Autodesk Inventor part; units mm, degrees
ref_plane "YZ Plane" through (0, 0, 0) normal (1, 0, 0) x (0, 1, 0)
ref_plane "XZ Plane" through (0, 0, 0) normal (0, 1, 0) x (-1, 0, 0)
ref_plane "XY Plane" through (0, 0, 0) normal (0, 0, 1) x (1, 0, 0)
sketch "Esquisse1" plane through (0, 0, 0) normal (0, 1, 0) x (-1, 0, 0)
  circle A0 centre (-0.3398, 0) radius 22.5
  circle A1 centre (-0.3398, 0) radius 10
  line L0 (3.1602, 9.3675) -> (-3.8398, 9.3675)
  line L1 (-3.8398, 9.3675) -> (-3.8398, 30.3675)
  line L2 (-3.8398, 30.3675) -> (3.1602, 30.3675)
  line L3 (3.1602, 30.3675) -> (3.1602, 9.3675)
  line L4 (-8.8398, 35.3675) -> (-8.8398, 4.3675)
  line L5 (-8.8398, 4.3675) -> (8.1602, 4.3675)
  line L6 (8.1602, 4.3675) -> (8.1602, 35.3675)
  line L7 (8.1602, 35.3675) -> (-8.8398, 35.3675)
  line L8 (17.1996, -3) -> (9.1996, -3)
  line L9 (9.1996, -3) -> (9.1996, 3)
  line L10 (9.1996, 3) -> (17.1996, 3)
  line L11 (17.1996, 3) -> (17.1996, -3)
  line L12 (15.5701, 15.9099) -> (-16.2497, -15.9099) construction
  line L13 (-0.3398, -15.9099) -> (-16.2497, -15.9099) construction
  line L14 (-16.2497, -15.9099) -> (-16.2497, 0) construction
  line L15 (-0.3398, -15.9099) -> (-0.3398, 0) construction
  line L16 (-0.3398, 0) -> (-16.2497, 0) construction
  circle A2 centre (-11.1699, -10.8301) radius 2.5
  line L17 (-11.1699, -10.8301) -> (-16.2497, -15.9099) construction
  line L18 (-7.4109, -7.0711) -> (-11.1699, -10.8301) construction
  point P0 (-8.8398, 20.8327)
  point P1 (8.1602, 20.8327)
  dimension "d2" = 45
  dimension "d3" = 20
  dimension "d4" = 7
  dimension "d5" = 21
  dimension "d6" = 5
  dimension "d7" = 6
  dimension "d8" = 8
  dimension "d9" = 5
extrude "Extrusion1" add sketch "Esquisse1" along normal blind 10 contours A0 L4 A1 L8 L11 L10 L6 | L6 A1 L3 A0 | A0 L3 L2 L1 L4 L7 L6 | A0 L1 A1 L4
chamfer "Chanfrein1" distance 2 distance2 1 1 edges at (13.6699, 0, -10.8301) measured on face at (8.7023, 6.6667, -11.2311)
properties part number "Pièce_maintient_pièce"
For this review, take the finished solid that the model builds, in its own axes (mm). A direction names the side the tool comes from. Coordinates: 2 decimals unless noted, no trailing zeros. Write each loop counter-clockwise with the first axis right and the second up, starting at its lowest first coordinate (ties: lowest second). Pieces come first, ordered by that corner, then holes. Notation, with made-up numbers: (35.5, 48.25) -> (51.5, 48.25) arc R19 ccw to (51.5, 61.25) -> close; hole circle Ø3 at (-14, 7). An arc over 180 degrees is marked (long way). Write each question's results on one line, items separated by ' | '. Start each with the question number.
1) Consider section C-C (y = 5.25). Write out the cut boundary in (x, z), plus the area to 3 significant figures.
2) Consider section A-A (z = 25.5). Write out the cut boundary in (x, y), plus the area to 3 significant figures.
3) Wall thickness on L1, parallel to X at y = 5.25, z = 0; L2, parallel to X at y = 1.5, z = 24; L3, parallel to Z at x = -12, y = 7.75: over which ranges is each line inside the solid? List them lowest first. Write a range as [from, to].
4) Consider section D-D (z = 32.5). Write out the cut boundary in (x, y).
5) The part is to be moulded in two halves that separate along Z. For faces 1 (the face through (-17.2, 5, 0)), 2 (the face through (-0.528, 4.93, -22.483)), 3 (the face through (11, 0, 0)), say which applies: +Z half, -Z half, draft (parallel to the pull), parting line (faces both ways), or undercut.
6) For faces 4 (the face through (0, 5, 30.368)), 5 (the face through (8.84, 5, 28)), 6 (the face through (-8.16, 5, 28)), list the 3-axis set-ups (+Z, -Z, +X, -X, +Y, -Y) from which the entire face can be reached by the end or side of a thin tool; tool diameter is ignored.
7) Insertion check: pin 1 (4 mm diameter, centred on y = 5.5, z = 6, fed in from -X); pin 2 (2 mm diameter, centred on x = 9.5, z = -8, fed in from -Y); pin 3 (18 mm diameter, centred on x = 0.34, z = 0, fed in from -Y); pin 4 (2 mm diameter, centred on y = 4.5, z = 20.5, fed in from -X). Each pin has a flat end and moves straight along its axis. Give the tip position at first contact, or say it passes through.
8) Consider section B-B (x = 5). Write out the cut boundary in (y, z).
Geometry says:
1) outline: (-8.16, 20.83) arc R22.5 ccw (long way) to (8.84, 20.83) -> (8.84, 35.37) -> (-8.16, 35.37) -> close; hole (-17.2, -3) -> (-9.2, -3) arc R10 ccw (long way) to (3.84, 9.37) -> (3.84, 30.37) -> (-3.16, 30.37) -> (-3.16, 9.37) arc R10 ccw to (-9.2, 3) -> (-17.2, 3) -> close; hole circle Ø5 at (11.17, -10.83) | area: 1,290 mm^2
2) outline: (-8.16, 0) -> (-3.16, 0) -> (-3.16, 10) -> (-8.16, 10) -> close; (3.84, 0) -> (8.84, 0) -> (8.84, 10) -> (3.84, 10) -> close | area: 100 mm^2
3) L1: [-22.16, -17.2], [10.34, 22.84] | L2: [-8.16, -3.16], [3.84, 8.84] | L3: [-18.81, -3], [3, 18.81]
4) outline: (-8.16, 0) -> (8.84, 0) -> (8.84, 10) -> (-8.16, 10) -> close
5) face 1: undercut | face 2: parting line | face 3: draft
6) face 4: +Y, -Y | face 5: +Z, +X, +Y, -Y | face 6: +Z, -X, +Y, -Y
7) pin 1: x = -21.8 | pin 2: y = 0 | pin 3: through | pin 4: x = -10.89
8) outline: (0, -22.01) -> (10, -22.01) -> (10, -8.85) -> (0, -8.85) -> close; (0, 8.85) -> (10, 8.85) -> (10, 35.37) -> (0, 35.37) -> close
